The listing builds one solid part. Answer for the finished solid, in the listing's coordinates (mm). Face numbers are marked on the shaded views. A direction names the side the tool comes from. Round coordinates to 2 decimals unless told otherwise and drop trailing zeros. Write each loop counter-clockwise with the first axis right and the second up, starting at its lowest first coordinate (ties: lowest second). Pieces come first, ordered by that corner, then holes. Notation, with made-up numbers: (-2.75, 58.25) - (56.25, 58.25) arc R27 cw to (56.25, 97.25) - close; hole circle Ø11 at (-23, 61.5). An arc over 180 degrees is marked (long way). Answer in a Markdown table with one row per item.
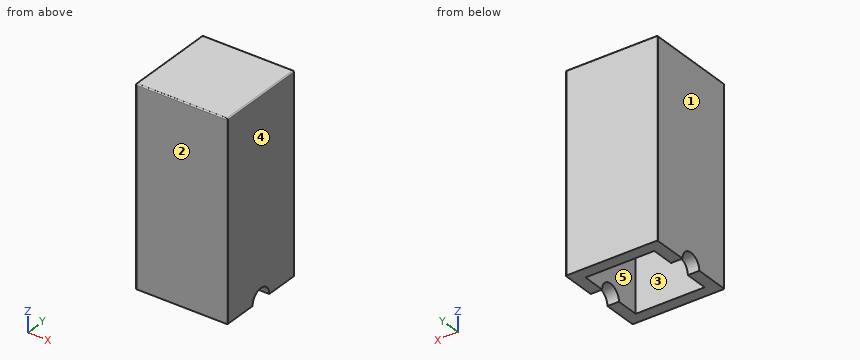
from build123d import *

# Parameters (mm, degrees)
F0_W     = 101.6
F0_H     = 101.6
F1_DEPTH = 215.9
F2_W     = 76.2
F2_H     = 76.2
F3_DEPTH = 162.56
F4_R     = 1.27
F5_R     = 12.7
F6_DEPTH = 101.601


with BuildPart() as f1:
    # F0 (on Top) → F1 (new body)
    with BuildSketch(Plane.XY):
        Rectangle(F0_W, F0_H)
    extrude(amount=F1_DEPTH)

    # F2 (on face) → F3 (cut)
    with BuildSketch(Plane(origin=(0, 0, 0), x_dir=(1, 0, 0), z_dir=(0, 0, -1))):
        Rectangle(F2_W, F2_H)
    extrude(amount=-F3_DEPTH, mode=Mode.SUBTRACT)

    # F4
    f4_edges = [f1.edges().sort_by_distance(p)[0] for p in [
        (50.8, -50.8, 107.95),
        (50.8, 0, 215.9),
        (50.8, 50.8, 107.95),
        (-50.8, -50.8, 107.95),
        (0, -50.8, 215.9),
        (0, 50.8, 215.9),
        (-50.8, 50.8, 107.95),
        (-50.8, 0, 215.9),
    ]]
    fillet(f4_edges, radius=F4_R)

    # F5 (on face) → F6 (cut, through all)
    with BuildSketch(Plane.YZ.offset(50.8)):
        Circle(F5_R)
    extrude(amount=-F6_DEPTH, mode=Mode.SUBTRACT)


solid = f1.part
(1) Find the intervals of material crossed by line 1 (X direction, y = 29.5, z = 17.5); line 2 (Z direction, x = 20, y = 16), in increasing order.
Checked values:
| item | result |
|---|---|
| line 1 | x = -50.8 to -38.1, 38.1 to 50.8 |
| line 2 | z = 162.56 to 215.9 |
(2) For a pull along Y with two mould halves and no side action, classify the marked faces 1, 2 and 3 as pulls with the +Y half, pulls with the -Y half, needs draft (parallel to the pull), parting line crosses it, or undercut.
Checked values:
| item | result |
|---|---|
| face 1 | needs draft |
| face 2 | pulls with the -Y half |
| face 3 | undercut |
(3) Section A-A (z = 134) is taken. Give the vertices of the cut face in (x, y).
Checked values:
| item | result |
|---|---|
| outline | (-50.8, -49.53) arc R1.27 ccw to (-49.53, -50.8) - (49.53, -50.8) arc R1.27 ccw to (50.8, -49.53) - (50.8, 49.53) arc R1.27 ccw to (49.53, 50.8) - (-49.53, 50.8) arc R1.27 ccw to (-50.8, 49.53) - close; hole (-38.1, -38.1) - (38.1, -38.1) - (38.1, 38.1) - (-38.1, 38.1) - close |
(4) A flat-ended cylindrical pin translates along its axis: pin 1 (1 mm diameter, centred on x = 29, y = -24.5, fed in from -Z). Find the tip coordinate at first contact, or state that the pin passes through.
Checked values:
| item | result |
|---|---|
| pin 1 | stops at z = 162.56 |
(5) Section B-B (y = -20.5) is taken. Give the vertices of the cut face in (x, z), and give its area (3 significant figures).
Checked values:
| item | result |
|---|---|
| outline | (-50.8, 0) - (-38.1, 0) - (-38.1, 162.56) - (38.1, 162.56) - (38.1, 0) - (50.8, 0) - (50.8, 214.63) arc R1.27 ccw to (49.53, 215.9) - (-49.53, 215.9) arc R1.27 ccw to (-50.8, 214.63) - close |
| area | 9,550 mm2 |
(6) For the marked faces 4 and 5, determine the directions among +Z, -Z, +X, -X, +Y, -Y from which every point of the face is accessible in a straight line to the end or side of a thin tool.
Checked values:
| item | result |
|---|---|
| face 4 | +Z, -Z, +X, +Y, -Y |
| face 5 | -Z |
